Verification items for this drawing (mm, ordinates from the low corner). A direction names the side the tool comes from. Round coordinates to 2 decimals unless told otherwise and drop trailing zeros. Write each loop counter-clockwise with the first axis right and the second up, starting at its lowest first coordinate (ties: lowest second). Pieces come first, ordered by that corner, then holes. Notation, with made-up numbers: (58, 64) -> (69, 64) arc R9 cw to (69, 77) -> close; hole circle Ø10 at (75, -8). An arc over 180 degrees is marked (long way). One line per question, with ' | ' between items.
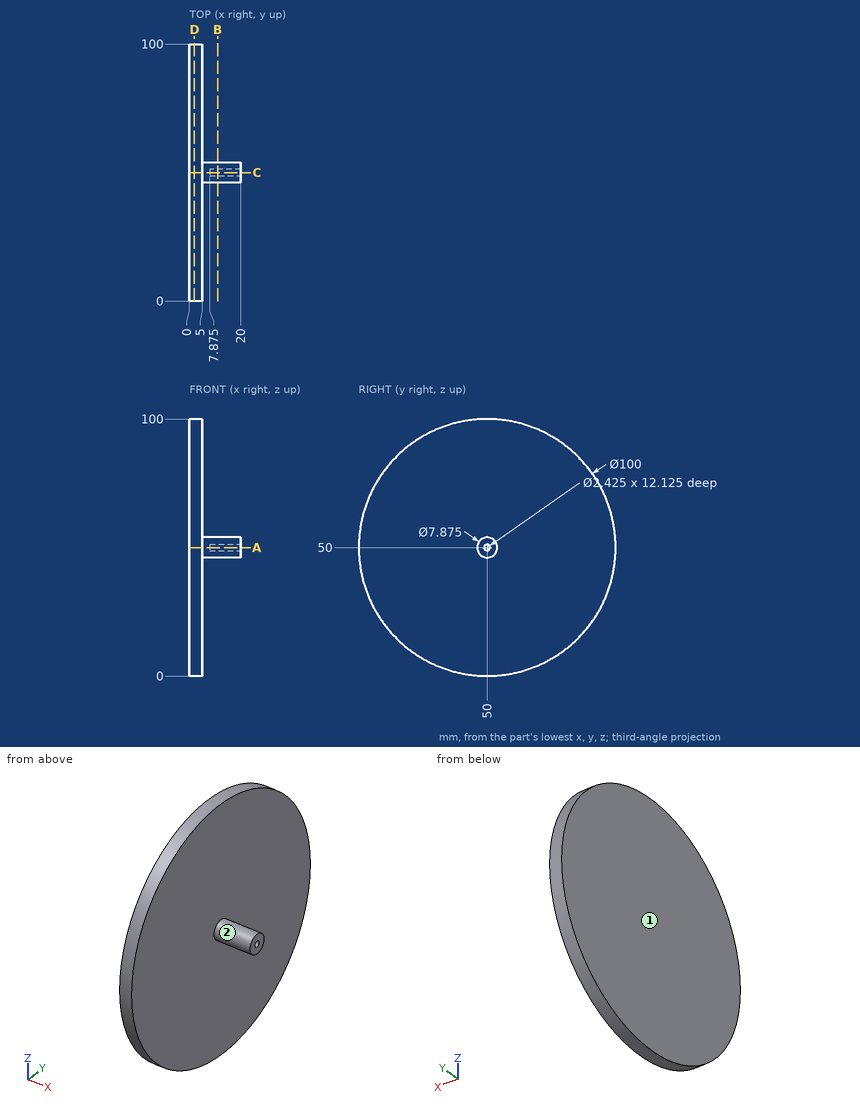
(1) Material ranges on line 1 (X direction, y = 62.5, z = 62); line 2 (Y direction, x = 18.25, z = 52); line 3 (Z direction, x = 3, y = 59), recorded low to high.
Resolved:
line 1: x = 0 to 5 | line 2: y = 46.61 to 53.39 | line 3: z = 0.82 to 99.18
(2) Sectioned sample at D-D on x = 2. Record the cut outline in (y, z).
Resolved:
outline: circle Ø100 at (50, 50)
(3) Sectioned sample at B-B on x = 11. Record the cut outline in (y, z) (1 decimal), then the cut area to 3 significant figures.
Resolved:
outline: circle Ø7.9 at (50, 50); hole circle Ø2.4 at (50, 50) | area: 44.1 mm2
(4) Sectioned sample at A-A on z = 50. Record the cut outline in (x, y) (1 decimal).
Resolved:
outline: (0, 0) -> (5, 0) -> (5, 46.1) -> (20, 46.1) -> (20, 48.8) -> (7.9, 48.8) -> (7.9, 51.2) -> (20, 51.2) -> (20, 53.9) -> (5, 53.9) -> (5, 100) -> (0, 100) -> close
(5) Access from +Z, -Z, +X, -X, +Y, -Y to the whole of each face (thin tool, end or side, straight path). Record for the marked faces 1 and 2.
Resolved:
face 1: +Z, -Z, -X, +Y, -Y | face 2: +X
(6) Go/stop test with flat-tipped pins: pin 1 (3 mm diameter, centred on x = 3.5, y = 35.5, fed in from +Z); pin 2 (6 mm diameter, centred on x = 7.5, y = 12.5, fed in from -Z); pin 3 (1.5 mm diameter, centred on x = 5, y = 33.5, fed in from -Z). Record where each tip stops, or that it passes through.
Resolved:
pin 1: stops at z = 98.28 | pin 2: stops at z = 15.14 | pin 3: stops at z = 2.55
